Work out the finished part from the listing and answer in its coordinate system (mm). A direction names the side the tool comes from. Give positions to 0.01 mm unless a question says otherwise; leave off trailing zeros. Loops run counter-clockwise (first coordinate to the right, second up) from the corner with the lowest first, then second, coordinate; pieces in that order, holes last. Notation, with made-up numbers: M 52.5,28 L 86.5,28 A10 ccw 86.5,38 Z; hole C 30,71.5 d6. An arc over 180 degrees is marked long. Answer as a JSON object with one key per item and string values. Group by question number.
```python
from build123d import *

# Parameters (mm, degrees)
BOX005_W          = 3
BOX005_H          = 9
BOX005_DEPTH      = 4
FILLET001_R       = 1
BOX003_W          = 10
BOX003_H          = 15
BOX003_DEPTH      = 4
FILLET003_R       = 1
BOX001_W          = 12.5
BOX001_H          = 15
BOX001_DEPTH      = 13
BOX_W             = 15
BOX_H             = 15
BOX_DEPTH         = 16
FILLET004_R       = 1
BOX004_W          = 4
BOX004_H          = 9
BOX004_DEPTH      = 3
FILLET_R          = 1
BOX002_W          = 4
BOX002_H          = 15
BOX002_DEPTH      = 10
FILLET002_R       = 1
FUSION_ROLL_ANGLE = 90


with BuildPart() as fillet001:
    # Box005 → Box005 (new body)
    with BuildSketch(Plane(origin=(18.5, 3, 0), x_dir=(1, 0, 0), z_dir=(0, 0, 1))):
        with Locations((1.5, 4.5)):
            Rectangle(BOX005_W, BOX005_H)
    extrude(amount=BOX005_DEPTH)

    # Fillet001
    fillet001_edges = [fillet001.edges().sort_by_distance(p)[0] for p in [
        (18.5, 3, 2),
        (18.5, 12, 2),
        (21.5, 3, 2),
        (21.5, 12, 2),
    ]]
    fillet(fillet001_edges, radius=FILLET001_R)


with BuildPart() as fillet003:
    # Box003 → Box003 (new body)
    with BuildSketch(Plane(origin=(15, 0, 0), x_dir=(1, 0, 0), z_dir=(0, 0, 1))):
        with Locations((5, 7.5)):
            Rectangle(BOX003_W, BOX003_H)
    extrude(amount=BOX003_DEPTH)

    # Cut002: cut Fillet001
    add(fillet001.part, mode=Mode.SUBTRACT)

    # Fillet003
    fillet003_edges = [fillet003.edges().sort_by_distance(p)[0] for p in [
        (25, 7.5, 4),
    ]]
    fillet(fillet003_edges, radius=FILLET003_R)


with BuildPart() as cube001:
    # Box001 → Box001 (new body)
    with BuildSketch(Plane(origin=(1.25, 0, 1.5), x_dir=(1, 0, 0), z_dir=(0, 0, 1))):
        with Locations((6.25, 7.5)):
            Rectangle(BOX001_W, BOX001_H)
    extrude(amount=BOX001_DEPTH)


with BuildPart() as fillet004:
    # Box → Box (new body)
    with BuildSketch(Plane.XY):
        with Locations((7.5, 7.5)):
            Rectangle(BOX_W, BOX_H)
    extrude(amount=BOX_DEPTH)

    # Cut: cut Cube001
    add(cube001.part, mode=Mode.SUBTRACT)

    # Fillet004
    fillet004_edges = [fillet004.edges().sort_by_distance(p)[0] for p in [
        (15, 7.5, 16),
    ]]
    fillet(fillet004_edges, radius=FILLET004_R)


with BuildPart() as fillet_body:
    # Box004 → Box004 (new body)
    with BuildSketch(Plane(origin=(0, 3, 19), x_dir=(1, 0, 0), z_dir=(0, 0, 1))):
        with Locations((2, 4.5)):
            Rectangle(BOX004_W, BOX004_H)
    extrude(amount=BOX004_DEPTH)

    # Fillet
    fillet_edges = [fillet_body.edges().sort_by_distance(p)[0] for p in [
        (2, 3, 19),
        (2, 3, 22),
        (2, 12, 19),
        (2, 12, 22),
    ]]
    fillet(fillet_edges, radius=FILLET_R)


with BuildPart() as fusion:
    # Box002 → Box002 (new body)
    with BuildSketch(Plane.XY.offset(16)):
        with Locations((2, 7.5)):
            Rectangle(BOX002_W, BOX002_H)
    extrude(amount=BOX002_DEPTH)

    # Cut001: cut Fillet body
    add(fillet_body.part, mode=Mode.SUBTRACT)

    # Fillet002
    fillet002_edges = [fusion.edges().sort_by_distance(p)[0] for p in [
        (4, 7.5, 26),
    ]]
    fillet(fillet002_edges, radius=FILLET002_R)

    # Fusion: union Fillet003, Fillet004
    add(fillet003.part)
    add(fillet004.part)


with BuildPart() as fusion_1:
    # Fusion roll: moved
    add(fusion.part.rotate(Axis((0, 0, 0), (1, 0, 0)), FUSION_ROLL_ANGLE))


with BuildPart() as fusion_2:
    # Fusion placement: moved
    add(fusion_1.part)


solid = fusion_2.part
```
Item 1: A cutting plane is placed at C-C (y = -8.75). Determine the outline of the cut face in (x, z), and give its area (3 significant figures).
Item 2: A tool of negligible diameter and unlimited length cuts with its end or side. For faces 5 (the cylindrical face through (21.215, -2.028, 11.699)), 6 (the flat face through (7, -14.5, 8)), 7 (the flat face through (4, -18, 7)), from which of +Z, -Z, +X, -X, +Y, -Y can it reach the whole face along a straight path? Write none if from no direction.
Item 3: A cutting plane is placed at D-D (z = 13.25). Determine the outline of the cut face in (x, y), and give its area (3 significant figures).
Item 4: A cutting plane is placed at B-B (x = 2.25). Determine the outline of the cut face in (y, z).
Item 5: Given pin 1 Ø5.5 at (y, z) = (-12, 8) entering from +X; pin 2 Ø3 at (x, z) = (8, 4) entering from -Y; pin 3 Ø3 at (x, y) = (17, -11) entering from +Z; pin 4 Ø7 at (y, z) = (-19, 5.5) entering from +X, each flat-ended and moving along its own axis, determine where each tip first touches the part or whether it passes through.
Item 6: For a pull along Y with two mould halves and no side action, classify faces 1 (the flat face through (9, -16, 8)), 2 (the cylindrical face through (2.028, -21.699, 11.715)), 3 (the flat face through (20, -2, 3)), 4 (the cylindrical face through (2.028, -21.699, 3.285)) as pulls with the +Y half, pulls with the -Y half, needs draft (parallel to the pull), parting line crosses it, or undercut.
Item 7: A cutting plane is placed at A-A (z = 10.5). Determine the outline of the cut face in (x, y).
Item 8: Find the intervals of material crossed by probe 1 along Y at (x, z) = (7, 9); probe 2 along X at (y, z) = (-13, 12.5); probe 3 along Y at (x, z) = (2.75, 5.25), in increasing order. Write a range as [from, to].
The answers:
{
 "1": {"outline": "M 0,0 L 1.25,0 L 1.25,15 L 0,15 Z; M 13.75,0 L 15,0 L 15,15 L 13.75,15 Z", "area": "37.5 mm^2"},
 "2": {"face 5": "+Y, -Y", "face 6": "+Z, -Z", "face 7": "+Z, -Z, +X, -Y"},
 "3": {"outline": "M 0,-26 L 3,-26 A1 ccw 4,-25 L 4,-16 L 14,-16 A1 ccw 15,-15 L 15,-4 L 24,-4 A1 ccw 25,-3 L 25,0 L 0,0 Z; hole M 1.25,-14.5 L 13.75,-14.5 L 13.75,-1.5 L 1.25,-1.5 Z", "area": "157 mm^2"},
 "4": {"outline": "M -26,0 L -14.5,0 L -14.5,15 L -26,15 Z; M -1.5,0 L 0,0 L 0,15 L -1.5,15 Z; hole M -22,4 A1 ccw -21,3 L -20,3 A1 ccw -19,4 L -19,11 A1 ccw -20,12 L -21,12 A1 ccw -22,11 Z"},
 "5": {"pin 1": "stops at x = 15", "pin 2": "stops at y = -16", "pin 3": "passes through", "pin 4": "stops at x = 14.87"},
 "6": {"face 1": "pulls with the -Y half", "face 2": "undercut", "face 3": "needs draft", "face 4": "undercut"},
 "7": {"outline": "M 0,-26 L 3,-26 A1 ccw 4,-25 L 4,-22 L 0,-22 Z; M 0,-19 L 4,-19 L 4,-16 L 14,-16 A1 ccw 15,-15 L 15,-4 L 18.5,-4 L 18.5,0 L 0,0 Z; M 21.5,-4 L 24,-4 A1 ccw 25,-3 L 25,0 L 21.5,0 Z; hole M 1.25,-14.5 L 13.75,-14.5 L 13.75,-1.5 L 1.25,-1.5 Z"},
 "8": {"probe 1": "y = [-16, -14.5], [-1.5, 0]", "probe 2": "x = [0, 1.25], [13.75, 15]", "probe 3": "y = [-26, -22], [-19, -14.5], [-1.5, 0]"}
}
